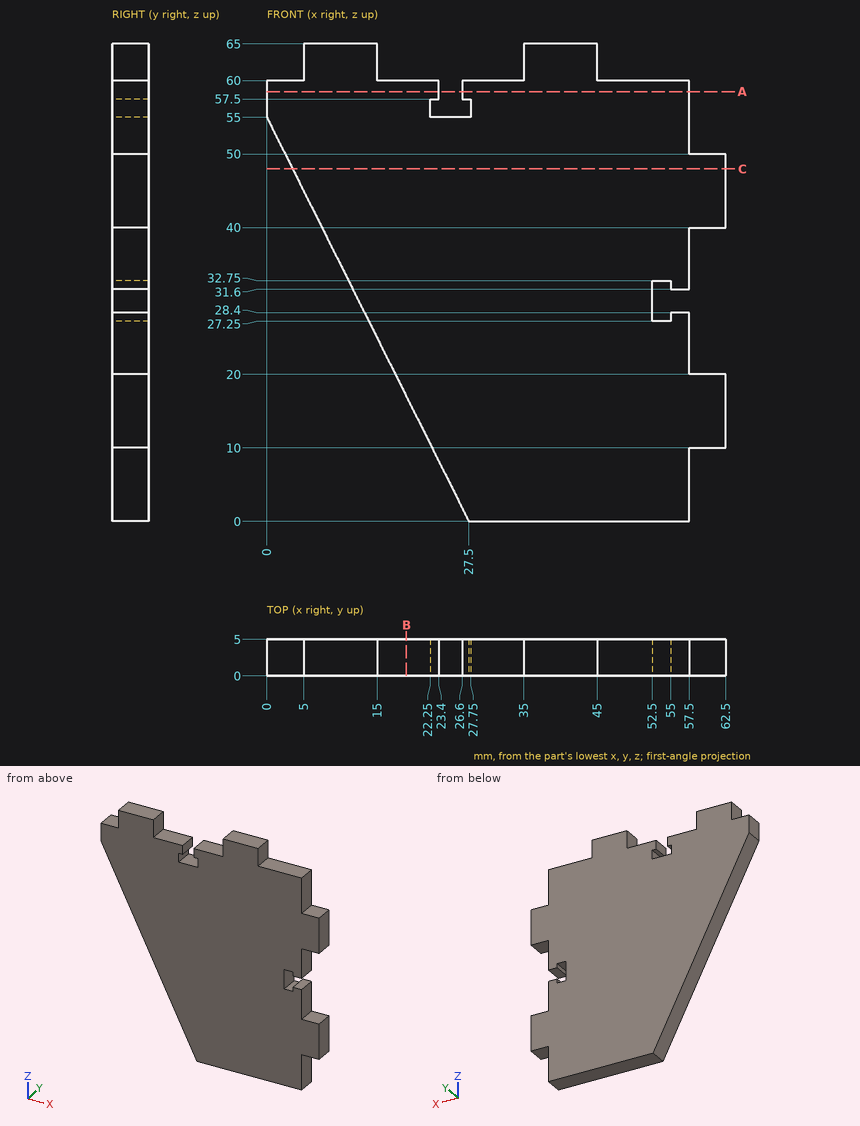
Can you work these out from the drawing? Everything is in mm from the part's minimum corner. Coordinates: 2 decimals unless noted, no trailing zeros. Loops run counter-clockwise (first coordinate to the right, second up) from the corner with the lowest first, then second, coordinate; pieces in that order, holes last. Notation, with made-up numbers: (60.25, -28.5) - (83.25, -28.5) arc R28 ccw to (83.25, -1.5) - close; hole circle Ø6 at (46.5, -13.5). An arc over 180 degrees is marked (long way). Use a Markdown table: item, result.
Item 1: I want a section at A-A on z = 58.5. Please give me the cut outline in (x, y).
Numbers:
| item | result |
|---|---|
| outline | (0, 0) - (23.4, 0) - (23.4, 5) - (0, 5) - close; (26.6, 0) - (57.5, 0) - (57.5, 5) - (26.6, 5) - close |
Item 2: Will these pins go through, and if not, where does the flat tip stop? pin 1 (2.5 mm diameter, centred on y = 2, z = 61.5, fed in from -X); pin 2 (2.5 mm diameter, centred on x = 26, y = 1.5, fed in from +Z); pin 3 (0.6 mm diameter, centred on x = 23, y = 2.5, fed in from -Z).
Numbers:
| item | result |
|---|---|
| pin 1 | stops at x = 5 |
| pin 2 | stops at z = 60 |
| pin 3 | stops at z = 8.4 |
Item 3: I want a section at C-C on z = 48. Please give me the cut outline in (x, y).
Numbers:
| item | result |
|---|---|
| outline | (3.5, 0) - (62.5, 0) - (62.5, 5) - (3.5, 5) - close |
Item 4: If I drill on probe 1 along Z at (x, y) = (58.5, 1.15); probe 2 along X at (y, z) = (4.4, 59.5); probe 3 along Z at (x, y) = (53, 0.95), over which ranges is the centre line in solid material (lowest first)? Write a range as from..to.
Numbers:
| item | result |
|---|---|
| probe 1 | z = 10..20, 40..50 |
| probe 2 | x = 0..23.4, 26.6..57.5 |
| probe 3 | z = 0..27.25, 32.75..60 |
Item 5: I want a section at B-B on x = 19. Please give me the cut outline in (y, z), and give its area (3 significant figures).
Numbers:
| item | result |
|---|---|
| outline | (0, 17) - (5, 17) - (5, 60) - (0, 60) - close |
| area | 215 mm2 |
